Work out the finished part from the listing and answer in its coordinate system (mm). Face numbers are marked on the shaded views. Give positions to 0.01 mm unless a question says otherwise; leave off trailing zeros. Loops run counter-clockwise (first coordinate to the right, second up) from the corner with the lowest first, then second, coordinate; pieces in that order, holes last. Notation, with made-up numbers: M 22.5,-27 L 28.5,-27 A4 ccw 28.5,-23 Z; hole C 36,-9 d4. An arc over 180 degrees is marked long. Use a Markdown table: item, result.
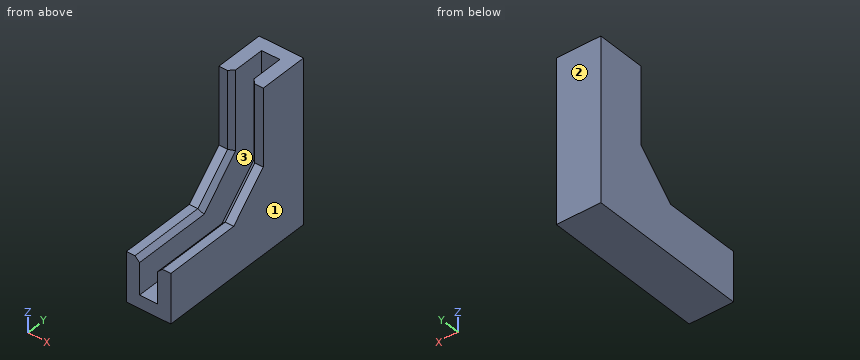
```python
from build123d import *

# Parameters (mm, degrees)
F3_SIZE = 8
F4_SIZE = 1


with BuildPart() as f2:
    # F2: sweep along a path in F0
    with BuildLine(Plane.YZ) as f2_path:
        Line((-25, 0), (0, 0))
        Line((0, 0), (0, 25))
    # F1 (on Front) → F2 (sweep)
    with BuildSketch(Plane.XZ):
        Polygon((-2, -8), (-2, 0), (-4.88, 0), (-4.88, -10.88), (4.88, -10.88), (4.88, 0), (2, 0), (2, -8), align=None)
    sweep(path=f2_path.line, transition=Transition.RIGHT)

    # F3
    f3_edges = [f2.edges().sort_by_distance(p)[0] for p in [
        (-3.44, 0, 0),
        (3.44, 0, 0),
    ]]
    chamfer(f3_edges, length=F3_SIZE)

    # F4
    f4_edges = [f2.edges().sort_by_distance(p)[0] for p in [
        (-2, -16.5, 0),
        (-2, 0, 16.5),
        (2, 0, 16.5),
        (2, -16.5, 0),
        (-2, -4, 4),
        (2, -4, 4),
    ]]
    chamfer(f4_edges, length=F4_SIZE)


solid = f2.part
```
(1) A cutting plane is placed at A-A (y = 6.5). Write down the section's boundary in (x, z).
Entries:
| item | result |
|---|---|
| outline | M -4.88,-10.88 L 4.88,-10.88 L 4.88,25 L 2,25 L 2,-8 L -2,-8 L -2,25 L -4.88,25 Z |
(2) A cutting plane is placed at B-B (z = -4). Write down the section's boundary in (x, y), and give its area (3 significant figures).
Entries:
| item | result |
|---|---|
| outline | M -4.88,-25 L -2,-25 L -2,8 L 2,8 L 2,-25 L 4.88,-25 L 4.88,10.88 L -4.88,10.88 Z |
| area | 218 mm² |
(3) A cutting plane is placed at D-D (y = -15). Write down the section's boundary in (x, z), and give its area (3 significant figures).
Entries:
| item | result |
|---|---|
| outline | M -4.88,-10.88 L 4.88,-10.88 L 4.88,0 L 3,0 L 2,-1 L 2,-8 L -2,-8 L -2,-1 L -3,0 L -4.88,0 Z |
| area | 73.2 mm² |
(4) A cutting plane is placed at C-C (x = -3.75). Write down the section's boundary in (y, z).
Entries:
| item | result |
|---|---|
| outline | M -25,-10.88 L 10.88,-10.88 L 10.88,25 L 0,25 L 0,8 L -8,0 L -25,0 Z |
(5) Consider probe 1 along X at (y, z) = (6, 16); probe 2 along Z at (x, y) = (-1, -3.5); probe 3 along Z at (x, y) = (-4.5, -6). Determine where each line is inside the solid, lowest interval first. Write a range as [from, to].
Entries:
| item | result |
|---|---|
| probe 1 | x = [-4.88, -2], [2, 4.88] |
| probe 2 | z = [-10.88, -8] |
| probe 3 | z = [-10.88, 2] |
(6) Given P1, Ø2, axis at x = 0, y = -16, coming from the +Z side; P2, Ø4.5, axis at x = 1, z = 14.5, coming from the -Y side; P3, Ø0.6, axis at x = 4.5, y = -15.5, coming from the +Z side, each flat-ended and moving along its own axis, determine where each tip first touches the part or whether it passes through.
Entries:
| item | result |
|---|---|
| P1 | stops at z = -8 |
| P2 | stops at y = 0 |
| P3 | stops at z = 0 |
(7) The mould has two halves that part along X. Classify the marked faces 1, 2 and 3: released by +X, released by -X, zero draft, split by the parting line, or undercut.
Entries:
| item | result |
|---|---|
| face 1 | released by +X |
| face 2 | zero draft |
| face 3 | undercut |
